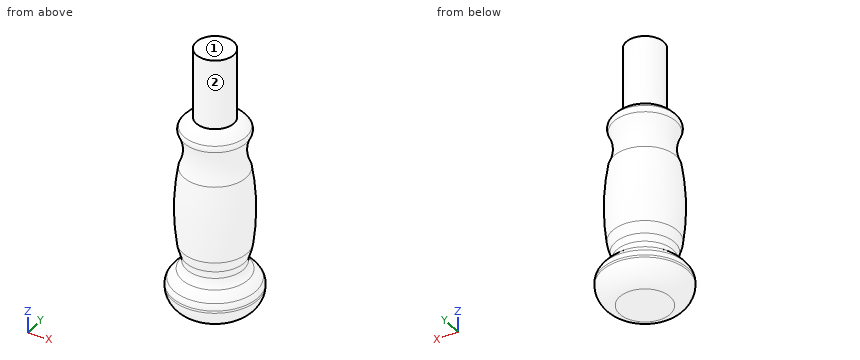
from build123d import *


with BuildPart() as part:
    # Sketch1 → Revolve5 (revolve)
    with BuildSketch(Plane(origin=(0, 0, 0), x_dir=(1, 0, 0), z_dir=(0, 1, 0))):
        with BuildLine():
            Line((-10.922, 0), (0, 0))
            Line((0, 0), (0, 152.4))
            Line((0, 152.4), (-14.648177892, 152.4))
            ThreePointArc((-14.648177892, 152.4), (-21.86995116, 148.183685931), (-24.9064291, 140.391952157))
            Line((-24.9064291, 140.391952157), (-24.9064291, 139.097981176))
            ThreePointArc((-24.9064291, 139.097981176), (-24.629788113, 137.189360348), (-23.822633993, 135.437827898))
            ThreePointArc((-23.822633993, 135.437827898), (-21.727400877, 132.742183052), (-19.206488947, 130.43968311))
            ThreePointArc((-19.206488947, 130.43968311), (-17.294597423, 128.178783744), (-16.491603127, 125.3288372))
            ThreePointArc((-16.491603127, 125.3288372), (-16.597847922, 123.122602782), (-17.179160796, 120.991679599))
            ThreePointArc((-17.179160796, 120.991679599), (-18.199132155, 117.877020277), (-18.845657016, 114.664007692))
            ThreePointArc((-18.845657016, 114.664007692), (-20.226314555, 92.4045447), (-18.146310091, 70.199511728))
            ThreePointArc((-18.146310091, 70.199511728), (-15.781686007, 59.957518133), (-18.146310091, 49.715524538))
            ThreePointArc((-18.146310091, 49.715524538), (-18.678899818, 47.821248891), (-18.146310091, 45.926973244))
            ThreePointArc((-18.146310091, 45.926973244), (-14.978108994, 42.676852004), (-10.922, 40.64))
            Line((-10.922, 40.64), (-10.922, 0))
        make_face()
    revolve(axis=Axis((0, 0, -152.4), (0, 0, 1)))


solid = part.part
For this review, take the finished solid that the model builds, in its own axes (mm). Face numbers are marked on the shaded views. A direction names the side the tool comes from. Round coordinates to 2 decimals unless told otherwise and drop trailing zeros. Loops run counter-clockwise (first coordinate to the right, second up) from the corner with the lowest first, then second, coordinate; pieces in that order, holes last. Notation, with made-up numbers: (-37, 87) - (-31, 87) arc R34 cw to (-31, 118) - close; hole circle Ø6 at (16, 30.5). An arc over 180 degrees is marked (long way). Answer as CSV lines item,"result".
(1) Wall thickness on line 1 (Y direction, x = 15, z = -135); line 2 (X direction, y = -4, z = -136); line 3 (X direction, y = 9, z = -26): over which ranges is each line inside the solid? List them lowest first.
Checked values:
line 1,"y = -18.13 to 18.13"
line 2,"x = -23.82 to 23.82"
line 3,"x = -6.19 to 6.19"
(2) Consider section A-A on z = -23.5. Give the boundary of the cut face in (x, y).
Checked values:
outline,"circle Ø21.84 at (0, 0)"
(3) Tool access review of the marked faces 1 and 2: name each direction out of +Z, -Z, +X, -X, +Y, -Y from which nothing blocks a thin tool from reaching the whole face with its end or side.
Checked values:
face 1,"+Z, +X, -X, +Y, -Y"
face 2,"+Z"
(4) Insertion check: P1, Ø6, axis at y = -5, z = -129, coming from the -X side; P2, Ø1.5, axis at y = 3.5, z = -121, coming from the +X side; P3, Ø12, axis at x = -3, y = 18, coming from the +Z side. Each pin has a flat end and moves straight along its axis. Give the tip position at first contact, or say it passes through.
Checked values:
P1,"stops at x = -20.48"
P2,"stops at x = 17.14"
P3,"stops at z = -41.12"
